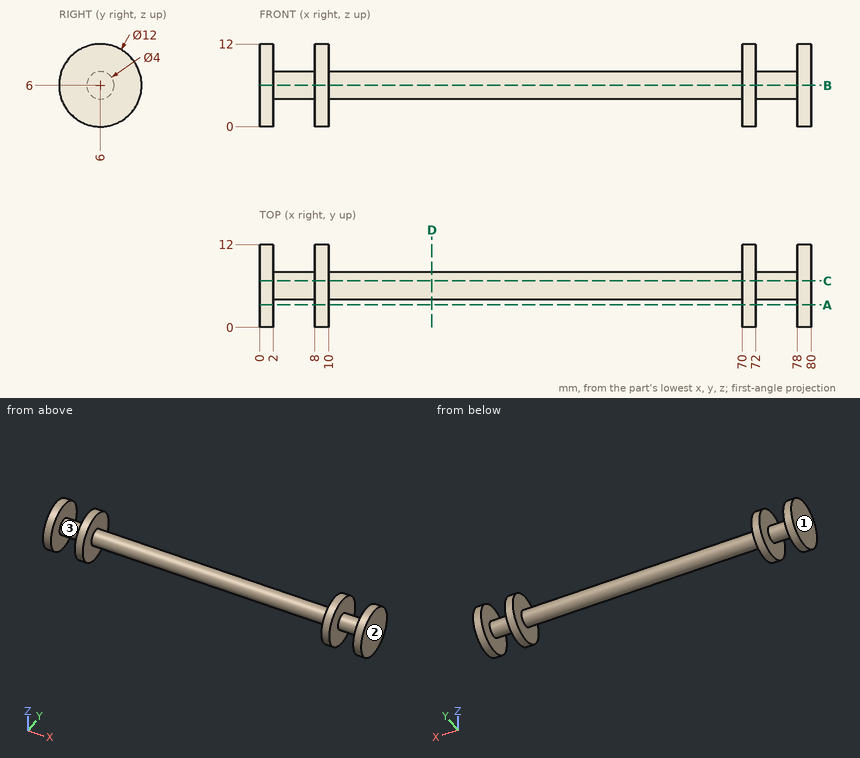
Study the drawing (mm; zero at the part's minimum x, y, z) and answer. Give positions to 0.01 mm unless a question says otherwise; leave off trailing zeros. Loops run counter-clockwise (first coordinate to the right, second up) from the corner with the lowest first, then second, coordinate; pieces in that order, holes last. Notation, with made-up numbers: (-6.75, -21.5) - (42.25, -21.5) arc R7 ccw to (42.25, -9.5) - close; hole circle Ø7 at (34.25, -10.75). An arc over 180 degrees is marked (long way). Return JSON: item names as keys, results as strings. Group by question number.
1. Find section A-A (y = 3.25). Write down the section's boundary in (x, z).
2. Determine the mould class of the marked faces 1, 2 and 3 for opening direction X: pulls with the +X half, pulls with the -X half, needs draft (parallel to the pull), parting line crosses it, or undercut.
3. Find section C-C (y = 6.75). Write down the section's boundary in (x, z), then the cut area to 3 significant figures.
4. Find section B-B (z = 6). Write down the section's boundary in (x, y).
5. Given pin 1 Ø6 at (x, y) = (54.5, 8.5) entering from +Z; pin 2 Ø1 at (x, z) = (49.5, 9.5) entering from +Y, each flat-ended and moving along its own axis, determine where each tip first touches the part or whether it passes through.
6. Find section D-D (x = 25). Write down the section's boundary in (y, z), then the cut area to 3 significant figures.
7. Straight lines are drawn through the part: line 1 (X direction, y = 6, z = 8.5); line 2 (Z direction, x = 61, y = 6.25); line 3 (Y direction, x = 20, z = 5.25). For each, find the intervals that lie inside material, in ascending order. Write a range as [from, to].
Verdict:
{
 "1": {"outline": "(0, 0.67) - (2, 0.67) - (2, 11.33) - (0, 11.33) - close; (8, 0.67) - (10, 0.67) - (10, 11.33) - (8, 11.33) - close; (70, 0.67) - (72, 0.67) - (72, 11.33) - (70, 11.33) - close; (78, 0.67) - (80, 0.67) - (80, 11.33) - (78, 11.33) - close"},
 "2": {"face 1": "pulls with the -X half", "face 2": "pulls with the +X half", "face 3": "undercut"},
 "3": {"outline": "(0, 0.05) - (2, 0.05) - (2, 4.15) - (8, 4.15) - (8, 0.05) - (10, 0.05) - (10, 4.15) - (70, 4.15) - (70, 0.05) - (72, 0.05) - (72, 4.15) - (78, 4.15) - (78, 0.05) - (80, 0.05) - (80, 11.95) - (78, 11.95) - (78, 7.85) - (72, 7.85) - (72, 11.95) - (70, 11.95) - (70, 7.85) - (10, 7.85) - (10, 11.95) - (8, 11.95) - (8, 7.85) - (2, 7.85) - (2, 11.95) - (0, 11.95) - close", "area": "362 mm^2"},
 "4": {"outline": "(0, 0) - (2, 0) - (2, 4) - (8, 4) - (8, 0) - (10, 0) - (10, 4) - (70, 4) - (70, 0) - (72, 0) - (72, 4) - (78, 4) - (78, 0) - (80, 0) - (80, 12) - (78, 12) - (78, 8) - (72, 8) - (72, 12) - (70, 12) - (70, 8) - (10, 8) - (10, 12) - (8, 12) - (8, 8) - (2, 8) - (2, 12) - (0, 12) - close"},
 "5": {"pin 1": "stops at z = 8", "pin 2": "passes through"},
 "6": {"outline": "circle Ø4 at (6, 6)", "area": "12.6 mm^2"},
 "7": {"line 1": "x = [0, 2], [8, 10], [70, 72], [78, 80]", "line 2": "z = [4.02, 7.98]", "line 3": "y = [4.15, 7.85]"}
}
